```python
from build123d import *

# Parameters (mm, degrees)
F0_W     = 50.8
F0_H     = 38.1
F1_DEPTH = 6.35
F2_R     = 14.2875
F3_DEPTH = 3.175
F4_R     = 1.397
F5_DEPTH = 6.35


with BuildPart() as f1:
    # F0 (on Top) → F1 (new body)
    with BuildSketch(Plane.XY):
        with Locations((25.4, 19.05)):
            Rectangle(F0_W, F0_H)
    extrude(amount=F1_DEPTH)

    # F2 (on face) → F3 (join)
    with BuildSketch(Plane.XY.offset(6.35)):
        with Locations((25.4, 19.05)):
            Circle(F2_R)
    extrude(amount=F3_DEPTH)

    # F4 (on face) → F5 (cut, through all)
    with BuildSketch(Plane.XY.offset(6.35)):
        with Locations((8.902216, 28.575)):
            Circle(F4_R)
        with Locations((41.897784, 28.575)):
            Circle(F4_R)
        with Locations((41.897784, 9.525)):
            Circle(F4_R)
        with Locations((8.902216, 9.525)):
            Circle(F4_R)
    extrude(amount=-F5_DEPTH, mode=Mode.SUBTRACT)


solid = f1.part
```
Geometry check sheet. Reference: the model listing, model coordinates, mm. A direction names the side the tool comes from. Coordinates: 2 decimals unless noted, no trailing zeros. Order: outer loops, then holes, each group sorted by start corner. A loop starts at its lowest first (then second) coordinate and runs counter-clockwise, first axis right, second up. Notation, with made-up numbers: (33.5, 49) - (55.5, 49) arc R30 ccw to (55.5, 82) - close; hole circle Ø7 at (-10.75, 83). An arc over 180 degrees is marked (long way). Answer in a Markdown table with one row per item. Add a question column.
1. Material ranges on L1, parallel to X at y = 28.5, z = 4.75; L2, parallel to Z at x = 38, y = 8; L3, parallel to Y at x = 27, z = 6.5, recorded low to high. Write a range as [from, to].
2. Section check D-D (x = 45). Enter the section's corners in (y, z), plus the area to 3 significant figures.
3. Gauge pin test, flat ends, axial feed: pin 1 Ø3 at (x, z) = (36.5, 8.5) entering from -Y; pin 2 Ø1.7 at (x, y) = (8.9, 9.52) entering from -Z; pin 3 Ø4.5 at (x, y) = (8.9, 28.58) entering from +Z. Record the tip position at first contact, or that the pin passes through.
4. Draft check along Y on faces 3 (the face through (25, 38.1, 3)), 4 (the face through (25, 19, 9.525)), 5 (the face through (41.72, 29.96, 3.22)). Enter one of: +Y half, -Y half, draft (parallel to the pull), parting line (faces both ways), or undercut.
5. Access from +Z, -Z, +X, -X, +Y, -Y to the whole of each face (thin tool, end or side, straight path). Record for faces 1 (the face through (25, 19, 0)), 2 (the face through (14.06, 10.36, 7.92)).
Data:
| question | item | result |
|---|---|---|
| 1 | L1 | x = [0, 7.51], [10.3, 40.5], [43.29, 50.8] |
| 1 | L2 | z = [0, 6.35] |
| 1 | L3 | y = [4.85, 33.25] |
| 2 | outline | (0, 0) - (38.1, 0) - (38.1, 6.35) - (0, 6.35) - close |
| 2 | area | 242 mm² |
| 3 | pin 1 | stops at y = 8.47 |
| 3 | pin 2 | passes through |
| 3 | pin 3 | stops at z = 6.35 |
| 4 | face 3 | +Y half |
| 4 | face 4 | draft |
| 4 | face 5 | undercut |
| 5 | face 1 | -Z, +X, -X, +Y, -Y |
| 5 | face 2 | +Z |
